Work out the finished part from the listing and answer in its coordinate system (mm). Face numbers are marked on the shaded views. Coordinates: 2 decimals unless noted, no trailing zeros. Loops run counter-clockwise (first coordinate to the right, second up) from the corner with the lowest first, then second, coordinate; pieces in that order, holes last. Notation, with made-up numbers: (48, 5) - (70, 5) arc R30 cw to (70, 40) - close; hole circle Ø5 at (31.5, 37.5). An arc over 180 degrees is marked (long way). Write each question's results on one line, items separated by ' | '. Start each with the question number.
Item 1: For a pull along X with two mould halves and no side action, classify the marked faces 1, 2 and 3 as +X half, -X half, draft (parallel to the pull), parting line (faces both ways), or undercut.
Item 2: Each of these flat-tipped pins is pushed along its axis until it touches: pin 1 Ø1.5 at (y, z) = (1.5, 7) entering from +X; pin 2 Ø1 at (x, y) = (-9.5, 1.5) entering from -Z; pin 3 Ø3 at (x, z) = (0, 0) entering from +Y. Where does it stop, or does it pass through?
Item 3: Section B-B, the plane x = 0 is taken. Write down the section's boundary in (y, z) (3 decimals).
Item 4: Section D-D, the plane z = 7.5 is taken. Write down the section's boundary in (x, y) (3 decimals), plus the area to 3 significant figures.
Item 5: Section C-C, the plane z = 0 is taken. Write down the section's boundary in (x, y) (3 decimals).
Item 6: Consider probe 1 along X at (y, z) = (2.3, 0); probe 2 along Z at (x, y) = (10.5, 2.85); probe 3 along X at (y, z) = (1.6, -8.5). Determine where each line is inside the solid, lowest interval first. Write a range as [from, to].
Item 7: Section A-A, the plane y = 2 is taken. Write down the section's boundary in (x, z).
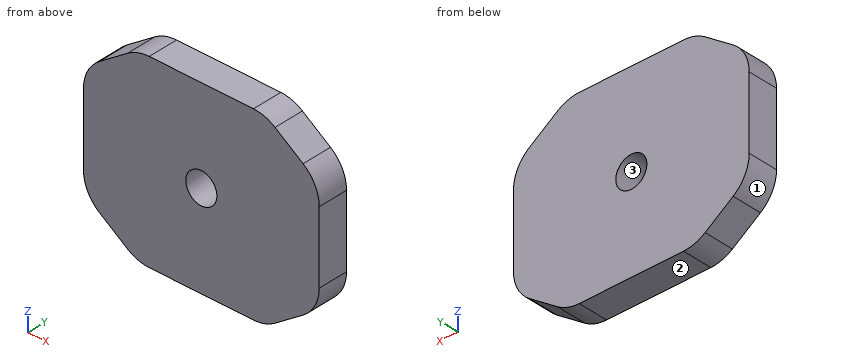
from build123d import *
from OCP.BRepFilletAPI import BRepFilletAPI_MakeChamfer

# Parameters (mm, degrees)
SKETCH2_W           = 25
SKETCH2_H           = 19.8
BOSS_EXTRUDE2_DEPTH = 3.175
SKETCH3_R           = 1.65
CUT_EXTRUDE1_DEPTH  = 3.175
CHAMFER1_SIZE       = 4
CHAMFER1_SIZE2      = 5.712592027
FILLET2_R           = 4


with BuildPart() as part:
    # Sketch2 → Boss-Extrude2 (new body)
    with BuildSketch(Plane(origin=(0, 0, 0), x_dir=(1, 0, 0), z_dir=(0, 1, 0))):
        Rectangle(SKETCH2_W, SKETCH2_H)
    extrude(amount=BOSS_EXTRUDE2_DEPTH)

    # Sketch3 → Cut-Extrude1 (cut)
    with BuildSketch(Plane(origin=(0, 3.175, 0), x_dir=(1, 0, 0), z_dir=(0, 1, 0))):
        with Locations(Location((0, 0, 0), (0, 0, 270))):
            Circle(SKETCH3_R)
    extrude(amount=-CUT_EXTRUDE1_DEPTH, mode=Mode.SUBTRACT)

    # Chamfer1: one chamfer whose edges measure the first distance from different faces: ONE call of the kernel's chamfer builder (chamfer() names one face for all edges)
    chamfer1_edges_1 = [part.edges().sort_by_distance(p)[0] for p in [
        (12.5, 1.5875, 9.9),
        (12.5, 1.5875, -9.9),
    ]]
    chamfer1_side_1 = [part.faces().sort_by_distance(p)[0] for p in [
        (12.5, 1.5875, 0),
    ]]
    chamfer1_edges_2 = [part.edges().sort_by_distance(p)[0] for p in [
        (-12.5, 1.5875, 9.9),
        (-12.5, 1.5875, -9.9),
    ]]
    chamfer1_side_2 = [part.faces().sort_by_distance(p)[0] for p in [
        (-12.5, 1.5875, 0),
    ]]
    chamfer1 = BRepFilletAPI_MakeChamfer(part.part.solid().wrapped)
    for e in chamfer1_edges_1:
        chamfer1.Add(CHAMFER1_SIZE, CHAMFER1_SIZE2, e.wrapped, chamfer1_side_1[0].wrapped)  # the first distance lies on this face
    for e in chamfer1_edges_2:
        chamfer1.Add(CHAMFER1_SIZE, CHAMFER1_SIZE2, e.wrapped, chamfer1_side_2[0].wrapped)  # the first distance lies on this face
    add(Compound.cast(chamfer1.Shape()), mode=Mode.REPLACE)

    # Fillet2
    fillet2_edges = [part.edges().sort_by_distance(p)[0] for p in [
        (12.5, 1.5875, -5.9),
        (12.5, 1.5875, 5.9),
        (-6.787407973, 1.5875, 9.9),
        (6.787407973, 1.5875, 9.9),
        (-12.5, 1.5875, -5.9),
        (-12.5, 1.5875, 5.9),
        (6.787407973, 1.5875, -9.9),
        (-6.787407973, 1.5875, -9.9),
    ]]
    fillet(fillet2_edges, radius=FILLET2_R)


solid = part.part
Answer key:
1) face 1: -X half | face 2: draft | face 3: undercut
2) pin 1: stops at x = 11.68 | pin 2: stops at z = -8.35 | pin 3: passes through
3) outline: (0, -9.9) - (3.175, -9.9) - (3.175, -1.65) - (0, -1.65) - close; (0, 1.65) - (3.175, 1.65) - (3.175, 9.9) - (0, 9.9) - close
4) outline: (-10.215, 0) - (10.215, 0) - (10.215, 3.175) - (-10.215, 3.175) - close | area: 64.9 mm^2
5) outline: (-12.5, 0) - (-1.65, 0) - (-1.65, 3.175) - (-12.5, 3.175) - close; (1.65, 0) - (12.5, 0) - (12.5, 3.175) - (1.65, 3.175) - close
6) probe 1: x = [-12.5, -1.65], [1.65, 12.5] | probe 2: z = [-7.3, 7.3] | probe 3: x = [-8.79, 8.79]
7) outline: (-12.5, -3.82) arc R4 ccw to (-10.79, -7.09) - (-7.82, -9.18) arc R4 ccw to (-5.53, -9.9) - (5.53, -9.9) arc R4 ccw to (7.82, -9.18) - (10.79, -7.09) arc R4 ccw to (12.5, -3.82) - (12.5, 3.82) arc R4 ccw to (10.79, 7.09) - (7.82, 9.18) arc R4 ccw to (5.53, 9.9) - (-5.53, 9.9) arc R4 ccw to (-7.82, 9.18) - (-10.79, 7.09) arc R4 ccw to (-12.5, 3.82) - close; hole circle Ø3.3 at (0, 0)
